from build123d import *

# Parameters (mm, degrees)
ESBO_O1_R                     = 4.25
RESSALTO_EXTRUS_O1_DEPTH      = 44
RESSALTO_EXTRUS_O2_DEPTH      = 6
RESSALTO_EXTRUS_O2_DEPTH_BACK = 50
ESBO_O2_R                     = 3.175
CHANFRO1_SIZE                 = 1
CHANFRO2_SIZE                 = 1


with BuildPart() as part:
    # Esboço1 → Ressalto-extrusão1 (new body)
    with BuildSketch(Plane(origin=(0, 0, 0), x_dir=(1, 0, 0), z_dir=(0, 1, 0))):
        with Locations(Location((0, 0, 0), (0, 0, 270))):
            Circle(ESBO_O1_R)
    extrude(amount=RESSALTO_EXTRUS_O1_DEPTH)

    # Esboço2 → Ressalto-extrusão2 (add, two sides: drawn at the far end of the back side and taken through both)
    with BuildSketch(Plane(origin=(0, 0, 0), x_dir=(-1, 0, 0), z_dir=(0, -1, 0)).offset(-RESSALTO_EXTRUS_O2_DEPTH_BACK)):
        with Locations(Location((0, 0, 0), (0, 0, 270))):
            Circle(ESBO_O2_R)
    extrude(amount=RESSALTO_EXTRUS_O2_DEPTH + RESSALTO_EXTRUS_O2_DEPTH_BACK)

    # Chanfro1
    chanfro1_edges = [part.edges().sort_by_distance(p)[0] for p in [
        (0, -6, -3.175),
    ]]
    chamfer(chanfro1_edges, length=CHANFRO1_SIZE)

    # Chanfro2
    chanfro2_edges = [part.edges().sort_by_distance(p)[0] for p in [
        (0, 50, -3.175),
    ]]
    chamfer(chanfro2_edges, length=CHANFRO2_SIZE)


solid = part.part
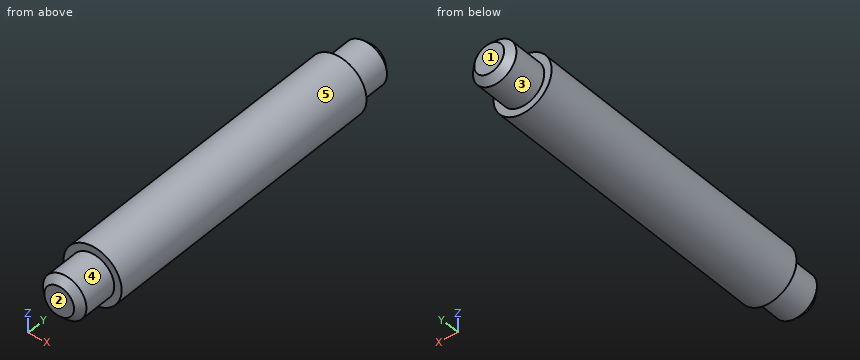
For this review, take the finished solid that the model builds, in its own axes (mm). Face numbers are marked on the shaded views. A direction names the side the tool comes from. Coordinates: 2 decimals unless noted, no trailing zeros. Order: outer loops, then holes, each group sorted by start corner. A loop starts at its lowest first (then second) coordinate and runs counter-clockwise, first axis right, second up. Notation, with made-up numbers: (68.5, -8.75) - (105.5, -8.75) arc R25 ccw to (105.5, 30.25) - close; hole circle Ø4 at (0, 82.25). An arc over 180 degrees is marked (long way). Answer as CSV lines item,"result". Start each with the question number.
1) Insertion check: P1, Ø4, axis at x = 2, y = 25.5, coming from the -Z side; P2, Ø1, axis at y = 15, z = 3, coming from the -X side; P3, Ø1.5, axis at x = 3, y = 17.5, coming from the +Z side; P4, Ø1, axis at x = -3, z = 3, coming from the +Y side. Each pin has a flat end and moves straight along its axis. Give the tip position at first contact, or say it passes through.
2) Add section A-A (x = 0). State the section outline as (y, z) points (3 decimals).
3) Draft analysis for pull direction Y (two halves, no side actions). For the marked faces 1, 2 and 3, state which applies: +Y half, -Y half, draft (parallel to the pull), parting line (faces both ways), or undercut.
4) Add section B-B (z = 0). State the section outline as (x, y) points (3 decimals), then the cut area to 3 significant figures.
5) Add section D-D (y = 46). State the section outline as (x, z) points (3 decimals), then the cut area to 3 significant figures.
6) To check wall thickness, follow line 1 along Y through (x, z) = (-3.5, 0); line 2 along Z through (x, y) = (0.25, 9); line 3 along X through (y, z) = (40.5, 2). State the ranges of each line that lie inside material, in increasing order. Write a range as [from, to].
7) Machinability: for the marked faces 4 and 5, which of the approach directions +Z, -Z, +X, -X, +Y, -Y give a long, thin tool a straight path to every point of the face, cutting with its end or side? Answer none if there is none.
8) Add section C-C (y = 10). State the section outline as (x, z) points.
Result:
1,P1,"z = -4.25"
1,P2,"x = -3.44"
1,P3,"z = 3.61"
1,P4,"y = 44"
2,outline,"(-6, -2.175) - (-5, -3.175) - (0, -3.175) - (0, -4.25) - (44, -4.25) - (44, -3.175) - (49, -3.175) - (50, -2.175) - (50, 2.175) - (49, 3.175) - (44, 3.175) - (44, 4.25) - (0, 4.25) - (0, 3.175) - (-5, 3.175) - (-6, 2.175) - close"
3,face 1,"+Y half"
3,face 2,"-Y half"
3,face 3,"draft"
4,outline,"(-4.25, 0) - (-3.175, 0) - (-3.175, -5) - (-2.175, -6) - (2.175, -6) - (3.175, -5) - (3.175, 0) - (4.25, 0) - (4.25, 44) - (3.175, 44) - (3.175, 49) - (2.175, 50) - (-2.175, 50) - (-3.175, 49) - (-3.175, 44) - (-4.25, 44) - close"
4,area,"448 mm^2"
5,outline,"circle Ø6.35 at (0, 0)"
5,area,"31.7 mm^2"
6,line 1,"[0, 44]"
6,line 2,"[-4.24, 4.24]"
6,line 3,"[-3.75, 3.75]"
7,face 4,"-Y"
7,face 5,"+Y, -Y"
8,outline,"circle Ø8.5 at (0, 0)"
